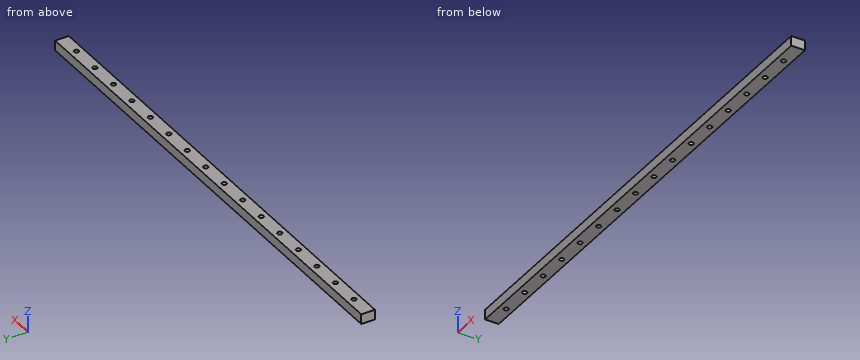
from build123d import *

# Parameters (mm, degrees)
SKETCH_W            = 331
SKETCH_H            = 9
PAD_DEPTH           = 6.5
SKETCH001_R         = 1.5
POCKET_DEPTH        = 6.501
LINEARPATTERN_COUNT = 16
LINEARPATTERN_PITCH = 20


with BuildPart() as part:
    # Sketch → Pad (new body)
    with BuildSketch(Plane.XY):
        with Locations((165.5, 4.5)):
            Rectangle(SKETCH_W, SKETCH_H)
    extrude(amount=PAD_DEPTH)

    # Sketch001 (on Face6 of Pad) → Pocket (cut, through all)
    with BuildSketch(Plane.XY.offset(6.5)):
        with Locations((15.4, 4.5)):
            Circle(SKETCH001_R)
    pocket = extrude(amount=-POCKET_DEPTH, mode=Mode.SUBTRACT)

    # LinearPattern: Pocket ×16
    with Locations(*[(i * LINEARPATTERN_PITCH, 0, 0) for i in range(1, LINEARPATTERN_COUNT)]):
        add(pocket, mode=Mode.SUBTRACT)


solid = part.part
Input: part model. Units: mm. Frame: model coordinates. Give positions to 0.01 mm unless a question says otherwise; leave off trailing zeros.
Q1. First-contact query: P1, Ø2.5, axis at x = 95.4, y = 4.5, coming from the -Z side. Flat tip, straight axial feed; report the tip coordinate or a pass-through.
Q2. Section A-A, the plane z = 2.25. State how many separate pieces and enclosed holes the cut face has, plus the area to 3 significant figures.
Q3. Material intervals for probe 1 along Y at (x, z) = (35.4, 3.5), sorted ascending.
Filled in:
1. P1: passes through
2. separate pieces: 1
2. enclosed holes: 16
2. area: 2,870 mm2
3. probe 1: y = 0 to 3, 6 to 9
